Verification items for the finished model (mm, model axes). Face numbers are marked on the shaded views. A direction names the side the tool comes from. Coordinates: 2 decimals unless noted, no trailing zeros. Write each loop counter-clockwise with the first axis right and the second up, starting at its lowest first coordinate (ties: lowest second). Pieces come first, ordered by that corner, then holes. Notation, with made-up numbers: (18.25, 58.5) -> (65.25, 58.5) arc R22 ccw to (65.25, 69.5) -> close; hole circle Ø3 at (17.25, 45.25). An arc over 180 degrees is marked (long way). Use a Markdown table: item, result. Add a question column.
from build123d import *

# Parameters (mm, degrees)
BOSS_EXTRUDE1_DEPTH = 16
SKETCH3_W           = 54
SKETCH3_H           = 5
BOSS_EXTRUDE2_DEPTH = 38
CUT_EXTRUDE4_DEPTH  = 10
SKETCH10_R          = 11
SKETCH10_R_2        = 7
BOSS_EXTRUDE4_DEPTH = 10
CUT_EXTRUDE5_DEPTH  = 10


with BuildPart() as part:
    # Sketch1 → Boss-Extrude1 (new, symmetric)
    with BuildSketch(Plane.XY):
        Polygon((0, 0), (54, 0), (54, -8), (31, -8), (31, -42), (23, -42), (23, -8), (0, -8), align=None)
    extrude(amount=BOSS_EXTRUDE1_DEPTH, both=True)

    # Sketch3 → Boss-Extrude2 (add)
    with BuildSketch(Plane(origin=(0, 0, 0), x_dir=(1, 0, 0), z_dir=(0, 1, 0))):
        with Locations((27, 13.5)):
            Rectangle(SKETCH3_W, SKETCH3_H)
    extrude(amount=BOSS_EXTRUDE2_DEPTH)

    # Sketch5 → Cut-Extrude4 (cut)
    with BuildSketch(Plane(origin=(0, 0, 0), x_dir=(1, 0, 0), z_dir=(0, 1, 0))):
        Polygon((44, -16), (54, -6), (54, -16), align=None)
        Polygon((10, -16), (0, -6), (0, -16), align=None)
    extrude(amount=-CUT_EXTRUDE4_DEPTH, mode=Mode.SUBTRACT)

    # Sketch10 → Boss-Extrude4 (add)
    with BuildSketch(Plane.XY.offset(-11)):
        with Locations(Location((27, 19, 0), (0, 0, 180))):
            Circle(SKETCH10_R)
        with Locations((27, 19)):
            Circle(SKETCH10_R_2, mode=Mode.SUBTRACT)
    extrude(amount=BOSS_EXTRUDE4_DEPTH)

    # Sketch12 → Cut-Extrude5 (cut)
    with BuildSketch(Plane.XY.offset(-11)):
        Polygon((0, 0), (10, 38), (0, 38), align=None)
        Polygon((44, 38), (54, 38), (54, 0), align=None)
    extrude(amount=-CUT_EXTRUDE5_DEPTH, mode=Mode.SUBTRACT)


solid = part.part
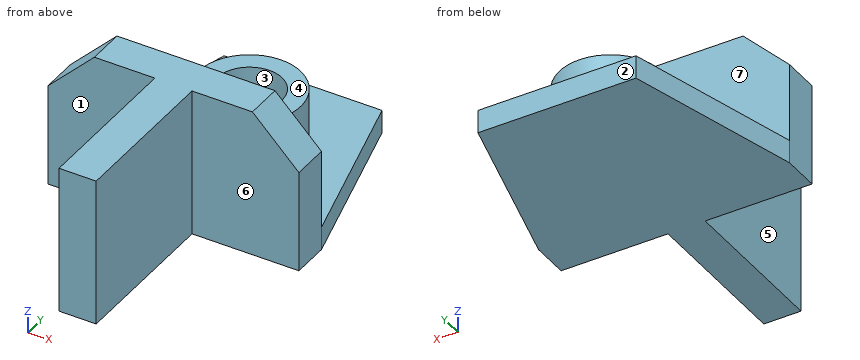
1) Set-up check for the marked faces 4, 5, 6 and 7: record each of +Z, -Z, +X, -X, +Y, -Y from which the full face is reachable in a straight line by a thin tool's end or side.
2) Cross-section at D-D on z = 4. Record the boundary of the cut face in (x, y).
3) Thickness scan on L1, parallel to Y at x = 27, z = -4; L2, parallel to Y at x = 25, z = -9; L3, parallel to Y at x = 35, z = 4. Record the ranges inside material, lowest first.
4) Cross-section at B-B on x = 27. Record the boundary of the cut face in (y, z).
5) Cross-section at A-A on z = -2. Record the boundary of the cut face in (x, y).
6) Gauge pin test, flat ends, axial feed: pin 1 (4 mm diameter, centred on y = 16, z = -7.5, fed in from +X); pin 2 (8 mm diameter, centred on x = 40.5, y = 21, fed in from +Z); pin 3 (18.5 mm diameter, centred on x = 12.5, z = 5.5, fed in from -Y); pin 4 (2 mm diameter, centred on x = 33.5, y = -10.5, fed in from -Z). Record the tip position at first contact, or that the pin passes through.
7) Cross-section at C-C on y = -1. Record the boundary of the cut face in (x, z), then the cut area to 3 significant figures.
8) Release check for a two-part mould opening along Y. For the marked faces 1, 2 and 3 record: released by +Y, released by -Y, zero draft, split by the parting line, or undercut.
Returned:
| question | item | result |
|---|---|---|
| 1 | face 4 | +Z, +X, -X, +Y |
| 1 | face 5 | +Z, -Z, -X, -Y |
| 1 | face 6 | +Z, -Z, +X, -Y |
| 1 | face 7 | +Z, +X, -X |
| 2 | outline | (0, -8) -> (23, -8) -> (23, -42) -> (31, -42) -> (31, -8) -> (54, -8) -> (54, 0) -> (0, 0) -> close |
| 3 | L1 | y = -42 to 0, 8 to 12, 26 to 30 |
| 3 | L2 | y = -42 to 0, 8.18 to 12.29, 25.71 to 29.82 |
| 3 | L3 | y = -8 to 0 |
| 4 | outline | (-42, -16) -> (38, -16) -> (38, -11) -> (30, -11) -> (30, -1) -> (26, -1) -> (26, -11) -> (12, -11) -> (12, -1) -> (8, -1) -> (8, -11) -> (0, -11) -> (0, 16) -> (-42, 16) -> close |
| 5 | outline | (0, -8) -> (23, -8) -> (23, -42) -> (31, -42) -> (31, -8) -> (54, -8) -> (54, 0) -> (0, 0) -> close; circle Ø22 at (27, 19); hole circle Ø14 at (27, 19) |
| 6 | pin 1 | stops at x = 37.95 |
| 6 | pin 2 | stops at z = -1 |
| 6 | pin 3 | stops at y = -8 |
| 6 | pin 4 | passes through |
| 7 | outline | (0, -16) -> (54, -16) -> (54, 6) -> (44, 16) -> (10, 16) -> (0, 6) -> close |
| 7 | area | 1,630 mm² |
| 8 | face 1 | released by -Y |
| 8 | face 2 | released by +Y |
| 8 | face 3 | undercut |
